```python
from build123d import *

# Parameters (mm, degrees)
SKETCH1_W           = 115
SKETCH1_H           = 115
BOSS_EXTRUDE2_DEPTH = 5
SKETCH3_W           = 129
SKETCH3_H           = 129
BOSS_EXTRUDE3_DEPTH = 35
SKETCH4_W           = 109
SKETCH4_H           = 109
CUT_EXTRUDE1_DEPTH  = 35
FILLET1_R           = 10
SKETCH6_W           = 109
SKETCH6_H           = 33
BOSS_EXTRUDE5_DEPTH = 50


with BuildPart() as part:
    # Sketch1 → Boss-Extrude2 (new body)
    with BuildSketch(Plane(origin=(0, 0, 0), x_dir=(1, 0, 0), z_dir=(0, 1, 0))):
        Rectangle(SKETCH1_W, SKETCH1_H)
    extrude(amount=BOSS_EXTRUDE2_DEPTH)

    # Sketch3 → Boss-Extrude3 (add)
    with BuildSketch(Plane.XZ):
        Rectangle(SKETCH3_W, SKETCH3_H)
    extrude(amount=BOSS_EXTRUDE3_DEPTH)

    # Sketch4 → Cut-Extrude1 (cut)
    with BuildSketch(Plane(origin=(0, 5, 0), x_dir=(1, 0, 0), z_dir=(0, 1, 0))):
        Rectangle(SKETCH4_W, SKETCH4_H)
    extrude(amount=-CUT_EXTRUDE1_DEPTH, mode=Mode.SUBTRACT)

    # Fillet1
    fillet1_edges = [part.edges().sort_by_distance(p)[0] for p in [
        (64.5, -17.5, -64.5),
        (64.5, -17.5, 64.5),
        (-64.5, -17.5, 64.5),
        (-64.5, -17.5, -64.5),
    ]]
    fillet(fillet1_edges, radius=FILLET1_R)

    # Sketch6 → Boss-Extrude5 (add)
    with BuildSketch(Plane(origin=(0, 0, 54.5), x_dir=(-1, 0, 0), z_dir=(0, 0, -1))):
        with Locations((0, -13.5)):
            Rectangle(SKETCH6_W, SKETCH6_H)
    extrude(amount=BOSS_EXTRUDE5_DEPTH)


solid = part.part
```
Could you check a few things on this model? Use its own coordinates, in mm. A direction names the side the tool comes from. Coordinates: 2 decimals unless noted, no trailing zeros. Order: outer loops, then holes, each group sorted by start corner. A loop starts at its lowest first (then second) coordinate and runs counter-clockwise, first axis right, second up. Notation, with made-up numbers: M 74.25,-9.5 L 129.25,-9.5 A27 ccw 129.25,10.5 Z; hole C 83,45.25 d5. An arc over 180 degrees is marked long. Use a Markdown table: item, result. Add a question column.
Q1. I want a section at A-A on z = -45.5. List the corners of the cut face in (x, y) for me.
Q2. We'd pull the mould along X, two halves only. Please class faces 1 (the flat face through (1, -13, 4.5)), 2 (the flat face through (64.5, -17, -1)), 3 (the flat face through (-64.5, -17, -1)), 4 (the flat face through (-1, -30, -25)): pulls with the +X half, pulls with the -X half, needs draft (parallel to the pull), parting line crosses it, or undercut.
Q3. I want a section at D-D on z = 16. List the corners of the cut face in (x, y) for me.
Q4. Which directions (+Z, -Z, +X, -X, +Y, -Y) give clear straight access to the entire face, cutting with the end or side of a thin tool? Please do faces 5 (the flat face through (57.5, 2, 1)), 6 (the flat face through (-57.5, 2, 1)), 7 (the flat face through (1, 3, 30)), 8 (the flat face through (-1, 2, -57.5)), 9 (the flat face through (-1, 2, 57.5)).
Q5. I want a section at C-C on x = 35.5. List the corners of the cut face in (y, z) for me, then the cut area to 4 significant figures.
Q6. If I drill on L1, parallel to Z at x = -46, y = -11.5; L2, parallel to X at y = -11, z = -14.5; L3, parallel to Z at x = -39, y = 1, over which ranges is the centre line in solid material (lowest first)?
Q7. I'm going to push flat-ended pins straight in: pin 1 (1 mm diameter, centred on x = 16.5, y = 4, fed in from -Z); pin 2 (1.5 mm diameter, centred on y = 2, z = -3, fed in from -X); pin 3 (10 mm diameter, centred on x = 18, z = -32.5, fed in from +Y); pin 4 (5.5 mm diameter, centred on x = 23.5, y = 2.5, fed in from +Z). Where does each tip first touch, or does it pass through?
Q8. I want a section at B-B on y = -12.5. List the corners of the cut face in (x, z) for me, then the cut area to 3 significant figures.
Checked values:
| question | item | result |
|---|---|---|
| 1 | outline | M -64.5,-35 L 64.5,-35 L 64.5,0 L 57.5,0 L 57.5,5 L 54.5,5 L 54.5,-30 L -54.5,-30 L -54.5,5 L -57.5,5 L -57.5,0 L -64.5,0 Z |
| 2 | face 1 | undercut |
| 2 | face 2 | pulls with the +X half |
| 2 | face 3 | pulls with the -X half |
| 2 | face 4 | undercut |
| 3 | outline | M -64.5,-35 L 64.5,-35 L 64.5,0 L 57.5,0 L 57.5,5 L 54.5,5 L 54.5,3 L -54.5,3 L -54.5,5 L -57.5,5 L -57.5,0 L -64.5,0 Z |
| 4 | face 5 | +Z, -Z, +X, +Y |
| 4 | face 6 | +Z, -Z, -X, +Y |
| 4 | face 7 | +Y |
| 4 | face 8 | -Z, +X, -X, +Y |
| 4 | face 9 | +Z, +X, -X, +Y |
| 5 | outline | M -35,-64.5 L 0,-64.5 L 0,-57.5 L 5,-57.5 L 5,-54.5 L -30,-54.5 L -30,4.5 L 3,4.5 L 3,54.5 L 5,54.5 L 5,57.5 L 0,57.5 L 0,64.5 L -35,64.5 Z |
| 5 | area | 2,925 mm² |
| 6 | L1 | -64.5 to -54.5, 4.5 to 64.5 |
| 6 | L2 | -64.5 to -54.5, 54.5 to 64.5 |
| 6 | L3 | -57.5 to -54.5, 4.5 to 57.5 |
| 7 | pin 1 | z = -57.5 |
| 7 | pin 2 | x = -57.5 |
| 7 | pin 3 | y = -30 |
| 7 | pin 4 | z = 64.5 |
| 8 | outline | M -64.5,-54.5 A10 ccw -54.5,-64.5 L 54.5,-64.5 A10 ccw 64.5,-54.5 L 64.5,54.5 A10 ccw 54.5,64.5 L -54.5,64.5 A10 ccw -64.5,54.5 Z; hole M -54.5,-54.5 L 54.5,-54.5 L 54.5,4.5 L -54.5,4.5 Z |
| 8 | area | 10,100 mm² |
